Check sheet for the modelled part. Datum: model origin and axes. Units: mm. A direction names the side the tool comes from. Give positions to 0.01 mm unless a question says otherwise; leave off trailing zeros. Loops run counter-clockwise (first coordinate to the right, second up) from the corner with the lowest first, then second, coordinate; pieces in that order, holes last. Notation, with made-up numbers: (73.25, -8.5) -> (88.25, -8.5) arc R15 cw to (88.25, 16.5) -> close; hole circle Ø6 at (44, -37). An arc over 180 degrees is marked (long way). Answer as CSV lines item,"result". Start each with the question number.
(1) Release check for a two-part mould opening along Y. For faces 3 (the face through (187.281, 30.967, 3.131)), 4 (the face through (-15.92, 27.77, 3.13)), 5 (the face through (187.369, -5.545, 3.131)) record: pulls with the +Y half, pulls with the -Y half, needs draft (parallel to the pull), parting line crosses it, or undercut.
(2) Gauge pin test, flat end, axial feed: pin 1 Ø6 at (x, y) = (5.5, 17) entering from -Z. Record the tip position at first contact, or that the pin passes through.
(3) Material ranges on line 1 (Y direction, x = 31.5, z = 1.5), recorded low to high. Write a range as from..to.
(4) Section check A-A on x = 139. Enter the section's corners in (y, z).
(5) Access from +Z, -Z, +X, -X, +Y, -Y to the whole of each face (thin tool, end or side, straight path). Record for faces 1 (the face through (87, -6.35, 3)), 2 (the face through (85, 25.4, 3)).
from build123d import *

# Parameters (mm, degrees)
SKETCH1_W           = 171.45
SKETCH1_H           = 25.4
BOSS_EXTRUDE1_DEPTH = 6.35


with BuildPart() as part:
    # Sketch1 → Boss-Extrude1 (new body)
    with BuildSketch(Plane.XY):
        Polygon((-12.7, -6.35), (-19.05, -4.7625), (-12.7, -3.175), (-19.05, -1.5875), (-12.7, 0), (-19.05, 1.5875), (-12.7, 3.175), (-19.05, 4.7625), (-12.7, 6.35), (-19.05, 7.9375), (-12.7, 9.525), (-19.05, 11.1125), (-12.7, 12.7), (-19.05, 14.2875), (-12.7, 15.875), (-19.05, 17.4625), (-12.7, 19.05), (-19.05, 20.6375), (-12.7, 22.225), (-19.05, 23.8125), (-12.7, 25.4), (-19.05, 26.9875), (-12.7, 28.575), (-19.05, 30.1625), (-12.7, 31.75), (184.15, 31.75), (190.5, 30.1625), (184.15, 28.575), (190.5, 26.9875), (184.15, 25.4), (190.5, 23.8125), (184.15, 22.225), (190.5, 20.6375), (184.15, 19.05), (190.5, 17.4625), (184.15, 15.875), (190.5, 14.2875), (184.15, 12.7), (190.5, 11.1125), (184.15, 9.525), (190.5, 7.9375), (184.15, 6.35), (190.5, 4.7625), (184.15, 3.175), (190.5, 1.5875), (184.15, 0), (190.5, -1.5875), (184.15, -3.175), (190.5, -4.7625), (184.15, -6.35), align=None)
        with Locations((85.725, 12.7)):
            Rectangle(SKETCH1_W, SKETCH1_H, mode=Mode.SUBTRACT)
    extrude(amount=BOSS_EXTRUDE1_DEPTH)


solid = part.part
Working result:
1,face 3,"pulls with the +Y half"
1,face 4,"undercut"
1,face 5,"pulls with the -Y half"
2,pin 1,"passes through"
3,line 1,"y = -6.35..0, 25.4..31.75"
4,outline,"(-6.35, 0) -> (0, 0) -> (0, 6.35) -> (-6.35, 6.35) -> close; (25.4, 0) -> (31.75, 0) -> (31.75, 6.35) -> (25.4, 6.35) -> close"
5,face 1,"+Z, -Z, +X, -X, -Y"
5,face 2,"+Z, -Z"
